from build123d import *

# Parameters (mm, degrees)
SKETCH1_R           = 1.4224
BOSS_EXTRUDE1_DEPTH = 3.175


with BuildPart() as part:
    # Sketch1 → Boss-Extrude1 (new body)
    with BuildSketch(Plane.XY):
        Polygon((5915.081902132, 2730.775703183), (5915.081902132, 2727.600703183), (5908.274702132, 2727.600703183), (5908.274702132, 2718.405903183), (6296.221602132, 2718.405903183), (6296.221602132, 2724.590803183), (6321.621602132, 2724.590803183), (6321.621602132, 2730.775703183), (6276.593752132, 2730.775703183), (6276.593752132, 2727.600703184), (6273.190152132, 2727.600703184), (6273.190152132, 2730.775703183), (6211.709452132, 2730.775703183), (6211.709452132, 2727.600703184), (6208.305852132, 2727.600703184), (6208.305852132, 2730.775703183), (6143.650152132, 2730.775703183), (6143.650152132, 2727.600703184), (6140.246552132, 2727.600703184), (6140.246552132, 2730.775703183), (6078.765852132, 2730.775703183), (6078.765852132, 2727.600703183), (6075.362252132, 2727.600703183), (6075.362252132, 2730.775703183), (6010.706552132, 2730.775703183), (6010.706552132, 2727.600703183), (6007.302952132, 2727.600703183), (6007.302952132, 2730.775703183), (5945.822252132, 2730.775703183), (5945.822252132, 2727.600703183), (5942.647252132, 2727.600703183), (5942.647252132, 2730.775703183), align=None)
        with Locations((5944.234752132, 2723.003303183)):
            Circle(SKETCH1_R, mode=Mode.SUBTRACT)
        with Locations((6009.119052132, 2723.003303183)):
            Circle(SKETCH1_R, mode=Mode.SUBTRACT)
        with Locations((6077.178352132, 2723.003303183)):
            Circle(SKETCH1_R, mode=Mode.SUBTRACT)
        with Locations((6142.062652132, 2723.003303183)):
            Circle(SKETCH1_R, mode=Mode.SUBTRACT)
        with Locations((6210.121952132, 2723.003303183)):
            Circle(SKETCH1_R, mode=Mode.SUBTRACT)
        with Locations((6275.006252132, 2723.003303183)):
            Circle(SKETCH1_R, mode=Mode.SUBTRACT)
        with Locations((5913.494402132, 2723.003303183)):
            Circle(SKETCH1_R, mode=Mode.SUBTRACT)
    extrude(amount=BOSS_EXTRUDE1_DEPTH)


solid = part.part
Model file for the job. Use its own axes, mm. Round coordinates to 2 decimals unless told otherwise and drop trailing zeros.
(1) Pin check, flat tips, straight feed: pin 1 (1 mm diameter, centred on x = 6210, z = 2.5, fed in from +Y); pin 2 (1 mm diameter, centred on y = 2721, z = 1.5, fed in from +X); pin 3 (1 mm diameter, centred on x = 6222, y = 2727.5, fed in from -Z). Stop position of each tip, or through.
(2) Band-saw the part on A-A (z = 1.3). Give the number of separate pieces and of enclosed holes in the cut face, then the cut area to 3 significant figures.
(3) Drill centre line: line 1 (X direction, y = 2721.25, z = 2.4). Where is it in solid material? Low to high.
Verdict:
1. pin 1: stops at y = 2727.6
1. pin 2: stops at x = 6296.22
1. pin 3: stops at z = 0
2. separate pieces: 1
2. enclosed holes: 7
2. area: 4,830 mm2
3. line 1: x = 5908.27 to 6296.22
